Design review of the part built by this model. Coordinates are the model's own, in mm. A direction names the side the tool comes from. Coordinates: 2 decimals unless noted, no trailing zeros. Loops run counter-clockwise (first coordinate to the right, second up) from the corner with the lowest first, then second, coordinate; pieces in that order, holes last. Notation, with made-up numbers: M 40.5,22.25 L 89.5,22.25 A26 cw 89.5,43.25 Z; hole C 39,14 d2. An arc over 180 degrees is marked long. Answer as CSV lines item,"result". Start each with the question number.
from build123d import *

# Parameters (mm, degrees)
ESQUISSE1_R        = 12.6
BOSS_EXTRU_1_DEPTH = 10
ESQUISSE2_R        = 6.4
BOSS_EXTRU_2_DEPTH = 9.7
D_GAGEMENT_M1_61_D = 2


with BuildPart() as part:
    # Esquisse1 → Boss.-Extru.1 (new body)
    with BuildSketch(Plane(origin=(0, 0, 0), x_dir=(1, 0, 0), z_dir=(0, 1, 0))):
        with Locations(Location((0, 0, 0), (0, 0, 270))):
            Circle(ESQUISSE1_R)
    extrude(amount=BOSS_EXTRU_1_DEPTH)

    # Esquisse2 → Boss.-Extru.2 (add)
    with BuildSketch(Plane(origin=(0, 10, 0), x_dir=(1, 0, 0), z_dir=(0, 1, 0))):
        with Locations(Location((0, 0, 0), (0, 0, 270))):
            Circle(ESQUISSE2_R)
    extrude(amount=BOSS_EXTRU_2_DEPTH)

    # Dégagement M1.61 (through all)
    with Locations(Plane(origin=(0, 19.7, 0), x_dir=(1, 0, 0), z_dir=(0, 1, 0))):
        with Locations((0, 0)):
            Hole(D_GAGEMENT_M1_61_D / 2)


solid = part.part
Item 1: Add section C-C (y = 12.25). Give the boundary of the cut face in (x, z).
Item 2: For pin 1 (3 mm diameter, centred on y = 15, z = -6.5, fed in from -X) (3 decimals); pin 2 (2 mm diameter, centred on x = 1, y = 13, fed in from -Z); pin 3 (3 mm diameter, centred on y = 16.5, z = -5, fed in from +X), all flat-tipped, find the tip position at first contact; note any pin that passes through.
Item 3: For line 1 along Y through (x, z) = (2.25, -6.5); line 2 along Z through (x, y) = (-0.75, 3.5); line 3 along X through (y, z) = (9.5, -0.25), list the stretches that pass through material, from the lowest coordinate up. Write a range as from..to.
Item 4: Add section A-A (x = 0). Give the boundary of the cut face in (y, z).
Item 5: Mouldability with a two-part tool opening along Z and no side actions: class faces 3 (the face through (0, 10, 1)), 4 (the face through (0.1, 19.7, 1.3)), 5 (the face through (-3.89, 14.78, -5.08)) as released by +Z, released by -Z, zero draft, split by the parting line, or undercut.
Item 6: Add section D-D (y = 7). Give the boundary of the cut face in (x, z), plus the area to 3 significant figures.
Item 7: For faces 1 (the face through (-7.667, 4.93, -9.999)), 2 (the face through (3, 10, -6)), list the 3-axis set-ups (+Z, -Z, +X, -X, +Y, -Y) from which the entire face can be reached by the end or side of a thin tool; tool diameter is ignored.
Item 8: Add section B-B (z = 0). Give the boundary of the cut face in (x, y).
Response:
1,outline,"C 0,0 d12.8; hole C 0,0 d2"
2,pin 1,"x = -3.995"
2,pin 2,"z = -6.4"
2,pin 3,"x = 5.36"
3,line 1,"0..10"
3,line 2,"-12.58..-0.66, 0.66..12.58"
3,line 3,"-12.6..-0.97, 0.97..12.6"
4,outline,"M 0,-12.6 L 10,-12.6 L 10,-6.4 L 19.7,-6.4 L 19.7,-1 L 0,-1 Z; M 0,1 L 19.7,1 L 19.7,6.4 L 10,6.4 L 10,12.6 L 0,12.6 Z"
5,face 3,"undercut"
5,face 4,"zero draft"
5,face 5,"split by the parting line"
6,outline,"C 0,0 d25.2; hole C 0,0 d2"
6,area,"496 mm²"
7,face 1,"+Y, -Y"
7,face 2,"+Y"
8,outline,"M -12.6,0 L -1,0 L -1,19.7 L -6.4,19.7 L -6.4,10 L -12.6,10 Z; M 1,0 L 12.6,0 L 12.6,10 L 6.4,10 L 6.4,19.7 L 1,19.7 Z"
